Geometry: final body of the model. Coordinates: model frame, mm. Coordinates: 2 decimals unless noted, no trailing zeros. Loops run counter-clockwise (first coordinate to the right, second up) from the corner with the lowest first, then second, coordinate; pieces in that order, holes last. Notation, with made-up numbers: (-31, 86) - (-15, 86) arc R8 cw to (-15, 99) - close; hole circle Ø6 at (45, 83). An arc over 180 degrees is marked (long way). Answer in a Markdown table with one row per item.
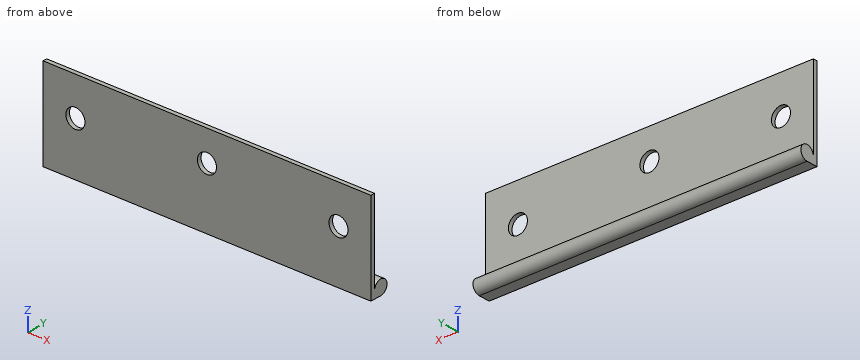
from build123d import *

# Parameters (mm, degrees)
SKETCH_1_R          = 1.9
EXTRUDE_1_DEPTH     = 86
SKETCH_2_R          = 2.5
CUT_EXTRUDE_1_DEPTH = 2.1


with BuildPart() as part:
    # 草图1 → 凸台-拉伸1 (new body)
    with BuildSketch(Plane(origin=(0, 0, 0), x_dir=(0, 0, -1), z_dir=(1, 0, 0))):
        with Locations((22, 3)):
            Circle(SKETCH_1_R)
        with BuildLine():
            Line((0, 1.1), (0, 0))
            Line((0, 0), (19, 0))
            Line((19, 0), (23.9, 0))
            Line((23.9, 0), (23.9, 3))
            ThreePointArc((23.9, 3), (23.343502884, 1.656497116), (22, 1.1))
            Line((22, 1.1), (19, 1.1))
            Line((19, 1.1), (0, 1.1))
        make_face()
    extrude(amount=EXTRUDE_1_DEPTH)

    # 草图2 → 切除-拉伸1 (cut, through all)
    with BuildSketch(Plane(origin=(0, 1.1, 0), x_dir=(1, 0, 0), z_dir=(0, 1, 0))):
        with Locations((8.5, 10)):
            Circle(SKETCH_2_R)
        with Locations((77.5, 10)):
            Circle(SKETCH_2_R)
        with Locations((43, 8)):
            Circle(SKETCH_2_R)
    extrude(amount=-CUT_EXTRUDE_1_DEPTH, mode=Mode.SUBTRACT)


solid = part.part
(1) Cut plane A-A on x = 8.5. Output: boundary loops of the cut face in (y, z).
Verdict:
| item | result |
|---|---|
| outline | (0, -23.9) - (3, -23.9) arc R1.9 ccw (long way) to (1.1, -22) - (1.1, -12.5) - (0, -12.5) - close; (0, -7.5) - (1.1, -7.5) - (1.1, 0) - (0, 0) - close |
(2) First-contact query: pin 1 Ø1 at (x, y) = (63, 2) entering from +Z; pin 2 Ø6 at (x, z) = (71.5, -11) entering from +Y. Flat tips, straight axial feed; report the tip coordinate or a pass-through.
Verdict:
| item | result |
|---|---|
| pin 1 | stops at z = -20.17 |
| pin 2 | stops at y = 1.1 |
(3) Ray query, probe 1 along Z at (x, y) = (43, 0.2); probe 2 along Z at (x, y) = (77.5, 0.9); probe 3 along X at (y, z) = (0.4, -10). Return the intervals inside material, ascending.
Verdict:
| item | result |
|---|---|
| probe 1 | z = -23.9 to -10.5, -5.5 to 0 |
| probe 2 | z = -23.9 to -12.5, -7.5 to 0 |
| probe 3 | x = 0 to 6, 11 to 41.5, 44.5 to 75, 80 to 86 |
(4) Cut plane B-B on z = -4.25. Output: boundary loops of the cut face in (x, y).
Verdict:
| item | result |
|---|---|
| outline | (0, 0) - (86, 0) - (86, 1.1) - (0, 1.1) - close |
